Geometry check sheet. Reference: the model listing, model coordinates, mm. A direction names the side the tool comes from. Give positions to 0.01 mm unless a question says otherwise; leave off trailing zeros. Write each loop counter-clockwise with the first axis right and the second up, starting at its lowest first coordinate (ties: lowest second). Pieces come first, ordered by that corner, then holes. Notation, with made-up numbers: (38.5, -36.5) -> (45.5, -36.5) arc R17 cw to (45.5, -19.5) -> close; hole circle Ø7 at (77.25, -26.75). An arc over 180 degrees is marked (long way). Write item = value, one per line. Start each with the question number.
1. Set-up check for faces 5 (the cylindrical face through (4.43, 9, -0.61)), 6 (the flat face through (5, 12, -7.8)): record each of +Z, -Z, +X, -X, +Y, -Y from which the full face is reachable in a straight line by a thin tool's end or side.
2. Cross-section at C-C, the plane y = 19.5. Record the cut outline in (x, z).
3. Cross-section at B-B, the plane x = 4.5. Record the cut outline in (y, z).
4. Mould release check, pull along Z, two halves, no side actions. Record for faces 1 (the cylindrical face through (8.392, 18.013, -4.305)), 2 (the flat face through (4, 12, 0)), 3 (the flat face through (9, 12, -4)), 4 (the flat face through (4, 12, -1.2)): pulls with the +Z half, pulls with the -Z half, needs draft (parallel to the pull), parting line crosses it, or undercut.
5. Cross-section at A-A, the plane z = -2. Record the cut outline in (x, y).
6. Thickness scan on line 1 along Z through (x, y) = (8.6, 19.5); line 2 along Z through (x, y) = (3.25, 21.5); line 3 along Y through (x, z) = (4.5, -0.4). Record the ranges inside material, lowest first.
7. Depth check by flat-ended pin: P1, Ø5, axis at y = 19.5, z = -4.5, coming from the +X side. Enter the tip coordinate at first touch or a pass-through.
8. Cross-section at D-D, the plane z = -4.5. Record the cut outline in (x, y).
Autodesk Inventor part; units mm, degrees
ref_plane "YZ Plane" through (0, 0, 0) normal (1, 0, 0) x (0, 1, 0)
ref_plane "XZ Plane" through (0, 0, 0) normal (0, 1, 0) x (-1, 0, 0)
ref_plane "XY Plane" through (0, 0, 0) normal (0, 0, 1) x (1, 0, 0)
sketch "スケッチ1" plane through (0, 0, 0) normal (0, 1, 0) x (-1, 0, 0)
  line L0 (0, 0) -> (-9, 0)
  line L1 (-9, 0) -> (-9, -9)
  line L2 (-9, -9) -> (0, -9)
  line L3 (0, -9) -> (0, 0)
  line L4 (-1.2, -1.2) -> (-7.8, -1.2)
  line L5 (-7.8, -1.2) -> (-7.8, -7.8)
  line L6 (-7.8, -7.8) -> (-1.2, -7.8)
  line L7 (-1.2, -7.8) -> (-1.2, -1.2)
  dimension "d0" = 9
  dimension "d1" = 9
  dimension "d2" = 6.6
  dimension "d3" = 6.6
  dimension "d4" = 1.2
  dimension "d5" = 1.2
extrude "押し出し1" add sketch "スケッチ1" along normal blind 24
sketch "スケッチ2" plane through (0, 0, 0) normal (0, 0, 1) x (1, 0, 0)
  line L0 (0, 0) -> (9, 0)
  line L1 (9, 0) -> (9, 24)
  point P0 (4.5, 7.5)
  dimension "d8" = 7.5
  dimension "d9" = 4.5
hole "穴1" at (4.5, 7.5, 0) direction (0, 0, -1) diameter 3 end through all
sketch "スケッチ3" plane through (9, 0, 0) normal (1, 0, 0) x (0, 0, -1)
  line L0 (0, 24) -> (9, 24)
  line L1 (9, 0) -> (9, 24)
  point P0 (0, 0)
  point P1 (4.5, 19.5)
  dimension "d17" = 4.5
  dimension "d18" = 4.5
hole "穴2" at (9, 19.5, -4.5) direction (-1, 0, 0) diameter 3 end through all
equation "\"d5\" = d4"
properties part number "前後直動9x9x24" material "アルミニウム 6061"
Answers:
q1.face_5 = +Z, -Z
q1.face_6 = +Y, -Y
q2.outline = (0, -9) -> (9, -9) -> (9, -6) -> (7.8, -6) -> (7.8, -7.8) -> (1.2, -7.8) -> (1.2, -6) -> (0, -6) -> close; (0, -3) -> (1.2, -3) -> (1.2, -1.2) -> (7.8, -1.2) -> (7.8, -3) -> (9, -3) -> (9, 0) -> (0, 0) -> close
q3.outline = (0, -9) -> (6, -9) -> (6, -7.8) -> (0, -7.8) -> close; (0, -1.2) -> (6, -1.2) -> (6, 0) -> (0, 0) -> close; (9, -9) -> (24, -9) -> (24, -7.8) -> (9, -7.8) -> close; (9, -1.2) -> (24, -1.2) -> (24, 0) -> (9, 0) -> close
q4.face_1 = undercut
q4.face_2 = pulls with the +Z half
q4.face_3 = needs draft
q4.face_4 = undercut
q5.outline = (0, 0) -> (1.2, 0) -> (1.2, 24) -> (0, 24) -> close; (7.8, 0) -> (9, 0) -> (9, 24) -> (7.8, 24) -> close
q6.line_1 = -9 to -6, -3 to 0
q6.line_2 = -9 to -7.8, -1.2 to 0
q6.line_3 = 0 to 6, 9 to 24
q7.P1 = 9
q8.outline = (0, 0) -> (1.2, 0) -> (1.2, 18) -> (0, 18) -> close; (0, 21) -> (1.2, 21) -> (1.2, 24) -> (0, 24) -> close; (7.8, 0) -> (9, 0) -> (9, 18) -> (7.8, 18) -> close; (7.8, 21) -> (9, 21) -> (9, 24) -> (7.8, 24) -> close
